Design review of the part built by this model. Coordinates are the model's own, in mm. A direction names the side the tool comes from. Coordinates: 2 decimals unless noted, no trailing zeros. Write each loop counter-clockwise with the first axis right and the second up, starting at its lowest first coordinate (ties: lowest second). Pieces come first, ordered by that corner, then holes. Notation, with made-up numbers: (73, 43) - (87, 43) arc R33 cw to (87, 78) - close; hole circle Ø10 at (-29.5, -11.75). An arc over 180 degrees is marked (long way). One line per item, written item: value.
from build123d import *

# Parameters (mm, degrees)
SKETCH1_R           = 7.5
BOSS_EXTRUDE2_DEPTH = 1.4
SKETCH3_R           = 9
SKETCH3_R_2         = 5
BOSS_EXTRUDE3_DEPTH = 1
FILLET1_R           = 3
SKETCH4_R           = 3.5
SKETCH4_R_2         = 2.5
BOSS_EXTRUDE5_DEPTH = 7
SKETCH5_R           = 2.5
CUT_EXTRUDE1_DEPTH  = 64.560554084


with BuildPart() as part:
    # Sketch1 → Boss-Extrude2 (new body)
    with BuildSketch(Plane(origin=(0, 2.1, 0), x_dir=(1, 0, 0), z_dir=(0, 1, 0))):
        with Locations(Location((-40.5, -30.5, 0), (0, 0, 270))):
            Circle(SKETCH1_R)
    extrude(amount=-BOSS_EXTRUDE2_DEPTH)

    # Sketch3 → Boss-Extrude3 (add)
    with BuildSketch(Plane(origin=(0, 2.1, 0), x_dir=(1, 0, 0), z_dir=(0, 1, 0))):
        with Locations(Location((-40.5, -30.5, 0), (0, 0, 270))):
            Circle(SKETCH3_R)
        with Locations(Location((-40.5, -30.5, 0), (0, 0, 270))):
            Circle(SKETCH3_R_2, mode=Mode.SUBTRACT)
    extrude(amount=BOSS_EXTRUDE3_DEPTH)

    # Fillet1
    # the kernel refuses this fillet: 3 mm, written as the material it adds along each edge
    with BuildSketch(Plane(origin=(-40.5, 2.1, 30.5), x_dir=(0, 0, 1), z_dir=(-1, 0, 0))) as fillet1_piece_1:
        with BuildLine():
            CenterArc((2.763932023, 3), FILLET1_R, 270, 48.189685104)
            Line((2.763932023, 0), (2.763932023, -0.06))
            Line((2.763932023, -0.06), (5, -0.06))
            Line((5, -0.06), (5.06, 0))
            ThreePointArc((5.06, 0), (5.06, 0.5), (5.04472136, 0.96))
            Line((5.04472136, 0.96), (5, 1))
        make_face()
    revolve(axis=Axis((-40.5, 2.1, 30.5), (0, 1, 0)))

    # Sketch4 → Boss-Extrude5 (add)
    with BuildSketch(Plane(origin=(-38.945196608, -1.435533906, 33.675308869), x_dir=(0.9504227777675709, 0.2313522039987804, -0.20778041583720402), z_dir=(-0.3109606783832559, 0.7071067811865516, -0.6350617737664737))):
        Circle(SKETCH4_R)
        with Locations(Location((0, 0, 0), (0, 0, 70.528842864))):
            Circle(SKETCH4_R_2, mode=Mode.SUBTRACT)
    extrude(amount=BOSS_EXTRUDE5_DEPTH)

    # Sketch5 → Cut-Extrude1 (cut, through all)
    with BuildSketch(Plane(origin=(3.199957151, -7.276519373, 6.535136451), x_dir=(0.9504227777675709, 0.2313522039987803, -0.20778041583720397), z_dir=(0.3109606783832558, -0.7071067811865516, 0.6350617737664735))):
        with Locations(Location((-44.343585554, 24.094947098, 0), (0, 0, 289.471157136))):
            Circle(SKETCH5_R)
    extrude(amount=-CUT_EXTRUDE1_DEPTH, mode=Mode.SUBTRACT)


solid = part.part
1. Mouldability with a two-part tool opening along Z and no side actions: class faces 1 (the face through (-47.82, 1.41, 28.87)), 2 (the face through (-39.54, 4.65, 32.7)), 3 (the face through (-44, 0.7, 30)) as released by +Z, released by -Z, zero draft, split by the parting line, or undercut.
Answer block:
face 1: split by the parting line
face 2: undercut
face 3: zero draft
2. For faces 4 (the face through (-40.47, -3.406, 32.228)), 5 (the face through (-33, 2.1, 28)), 6 (the face through (-44.4, 3.1, 34.4)), list the 3-axis set-ups (+Z, -Z, +X, -X, +Y, -Y) from which the entire face can be reached by the end or side of a thin tool; tool diameter is ignored.
Answer block:
face 4: +Z, +X, -Y
face 5: -Y
face 6: +Y
3. Insertion check: pin 1 Ø6 at (x, z) = (-37.5, 36.5) entering from -Y; pin 2 Ø4 at (x, y) = (-38.5, 1.5) entering from -Z; pin 3 Ø1 at (x, z) = (-43.5, 31.5) entering from -Y; pin 4 Ø5 at (x, z) = (-46.5, 26.5) entering from +Y. Each pin has a flat end and moves straight along its axis. Give the tip position at first contact, or say it passes through.
Answer block:
pin 1: stops at y = -0.47
pin 2: stops at z = 21.5
pin 3: stops at y = -0.88
pin 4: stops at y = 3.1
4. Wall thickness on line 1 along Z through (x, y) = (-41.5, 3); line 2 along Z through (x, y) = (-38.5, 2.75); line 3 along Y through (x, z) = (-34.5, 33): over which ranges is each line inside the solid? List them lowest first.
Answer block:
line 1: z = 21.56 to 25.7, 32.65 to 33.97, 35.3 to 39.44
line 2: z = 21.73 to 26.33, 27.1 to 28.9, 32.44 to 34.3, 34.67 to 39.27
line 3: y = 0.7 to 3.1
5. Consider section A-A, the plane x = -33.25. Write out the cut boundary in (y, z).
Answer block:
outline: (0.7, 28.58) - (2.1, 28.58) - (2.1, 25.17) - (3.1, 25.17) - (3.1, 35.83) - (2.1, 35.83) - (2.1, 32.42) - (0.7, 32.42) - close
6. Consider section B-B, the plane z = 37.5. Write out the cut boundary in (x, y).
Answer block:
outline: (-46.16, 2.1) - (-43.19, 2.1) - (-43.19, 0.7) - (-37.81, 0.7) - (-37.81, 2.1) - (-34.84, 2.1) - (-34.84, 3.1) - (-46.16, 3.1) - close
